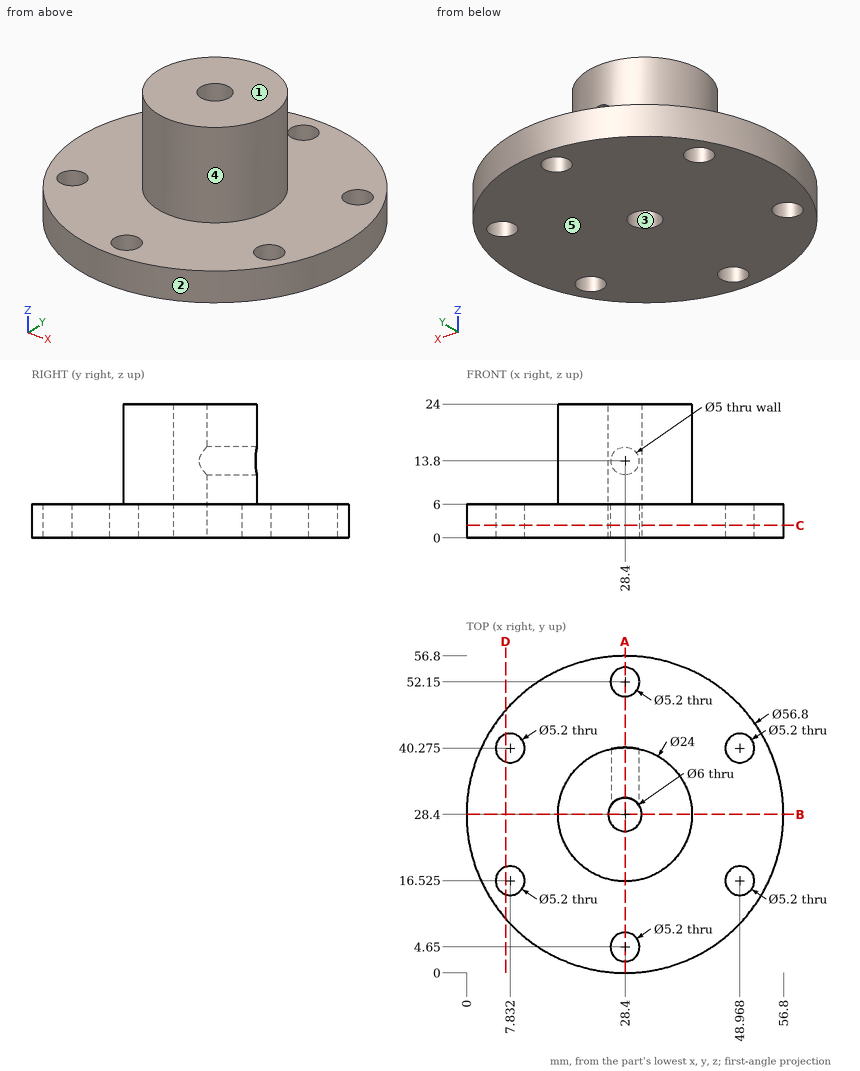
The drawing under review shows one solid part. Ordinate dimensions are in mm from its lowest x, y, z. A direction names the side the tool comes from. Round coordinates to 2 decimals unless told otherwise and drop trailing zeros. Write each loop counter-clockwise with the first axis right and the second up, starting at its lowest first coordinate (ties: lowest second). Pieces come first, ordered by that corner, then holes. Notation, with made-up numbers: (87, 18) - (97, 18) arc R32 cw to (97, 48) - close; hole circle Ø9 at (-31.5, -37.75). An arc over 180 degrees is marked (long way). Write each question's results on one line, items separated by ' | '.
Item 1: Take a section at B-B on y = 28.4. State the section outline as (x, z) points.
Calculated:
outline: (0, 0) - (25.4, 0) - (25.4, 24) - (16.4, 24) - (16.4, 6) - (0, 6) - close; (31.4, 0) - (56.8, 0) - (56.8, 6) - (40.4, 6) - (40.4, 24) - (31.4, 24) - close
Item 2: For the marked faces 4 and 5, list the 3-axis set-ups (+Z, -Z, +X, -X, +Y, -Y) from which the entire face can be reached by the end or side of a thin tool; tool diameter is ignored.
Calculated:
face 4: +Z | face 5: -Z, +X, -X, +Y, -Y
Item 3: To check wall thickness, follow line 1 along Y through (x, z) = (28.4, 2.2); line 2 along Y through (x, z) = (27.5, 4.5); line 3 along X through (y, z) = (18, 5.25). State the ranges of each line that lie inside material, in increasing order. Write a range as from..to.
Calculated:
line 1: y = 0..2.05, 7.25..25.4, 31.4..49.55, 54.75..56.8 | line 2: y = 0.01..2.21, 7.09..25.54, 31.26..49.71, 54.59..56.79 | line 3: x = 1.97..5.69, 9.97..46.83, 51.11..54.83
Item 4: Draft analysis for pull direction Y (two halves, no side actions). For the marked faces 1, 2 and 3, state which applies: pulls with the +Y half, pulls with the -Y half, needs draft (parallel to the pull), parting line crosses it, or undercut.
Calculated:
face 1: needs draft | face 2: parting line crosses it | face 3: undercut
Item 5: Take a section at D-D on x = 7. State the section outline as (y, z) points, then the cut area to 3 significant figures.
Calculated:
outline: (9.73, 0) - (14.06, 0) - (14.06, 6) - (9.73, 6) - close; (18.99, 0) - (37.81, 0) - (37.81, 6) - (18.99, 6) - close; (42.74, 0) - (47.07, 0) - (47.07, 6) - (42.74, 6) - close | area: 165 mm^2
Item 6: Take a section at C-C on z = 2.25. State the section outline as (x, y) points (3 decimals).
Calculated:
outline: circle Ø56.8 at (28.4, 28.4); hole circle Ø5.2 at (7.832, 16.525); hole circle Ø5.2 at (7.832, 40.275); hole circle Ø6 at (28.4, 28.4); hole circle Ø5.2 at (28.4, 4.65); hole circle Ø5.2 at (28.4, 52.15); hole circle Ø5.2 at (48.968, 16.525); hole circle Ø5.2 at (48.968, 40.275)
Item 7: Take a section at A-A on x = 28.4. State the section outline as (y, z) points.
Calculated:
outline: (0, 0) - (2.05, 0) - (2.05, 6) - (0, 6) - close; (7.25, 0) - (25.4, 0) - (25.4, 24) - (16.4, 24) - (16.4, 6) - (7.25, 6) - close; (31.4, 0) - (49.55, 0) - (49.55, 6) - (40.4, 6) - (40.4, 11.3) - (31.4, 11.3) - close; (31.4, 16.3) - (40.4, 16.3) - (40.4, 24) - (31.4, 24) - close; (54.75, 0) - (56.8, 0) - (56.8, 6) - (54.75, 6) - close
Item 8: For pin 1 (10 mm diameter, centred on x = 39.5, z = 17.5, fed in from -Y); pin 2 (6 mm diameter, centred on x = 48.97, y = 16.52, fed in from +Z); pin 3 (6 mm diameter, centred on x = 28.4, z = 13.8, fed in from -Y), all flat-tipped, find the tip position at first contact; note any pin that passes through.
Calculated:
pin 1: stops at y = 18.07 | pin 2: stops at z = 6 | pin 3: stops at y = 16.4
